Work out the finished part from the listing and answer in its coordinate system (mm). Coordinates: 2 decimals unless noted, no trailing zeros. Use one line per item in the form item = value.
from build123d import *

# Parameters (mm, degrees)
SKETCH_1_W      = 100
SKETCH_1_H      = 95
EXTRUDE_1_DEPTH = 2
HOLE_WIZARD_1_D = 3
FILLET_1_R      = 2


with BuildPart() as part:
    # 草图1 → 凸台-拉伸1 (new body)
    with BuildSketch(Plane(origin=(0, 0, 0), x_dir=(1, 0, 0), z_dir=(0, 1, 0))):
        Rectangle(SKETCH_1_W, SKETCH_1_H)
    extrude(amount=EXTRUDE_1_DEPTH)

    # 孔1 (through all)
    with Locations(Plane(origin=(0, 2, 0), x_dir=(1, 0, 0), z_dir=(0, 1, 0))):
        with Locations((-45, -12.906), (-42.5, 16.216), (42.673, 16.216), (45, -12.784)):
            Hole(HOLE_WIZARD_1_D / 2)

    # 圆角1
    fillet_1_edges = [part.edges().sort_by_distance(p)[0] for p in [
        (50, 1, 47.5),
        (-50, 1, 47.5),
        (-50, 1, -47.5),
        (50, 1, -47.5),
    ]]
    fillet(fillet_1_edges, radius=FILLET_1_R)


solid = part.part
(1) The mould has two halves that part along X. Classify faces 1 (the cylindrical face through (46.5, 0.99, 12.72)), 2 (the flat face through (-1, 0, -1)): released by +X, released by -X, zero draft, split by the parting line, or undercut.
Data:
face_1 = undercut
face_2 = zero draft
(2) Straight lines are drawn through the part: line 1 along X through (y, z) = (1.15, -16); line 2 along Z through (x, y) = (45, 0.5); line 3 along X through (y, z) = (0.5, 14). For each, find the intervals that lie inside material, in ascending order.
Data:
line_1 = -50 to -43.98, -41.02 to 41.19, 44.16 to 50
line_2 = -47.5 to 11.28, 14.28 to 47.5
line_3 = -50 to -46.03, -43.97 to 44.12, 45.88 to 50
(3) Each of these flat-tipped pins is pushed along its axis until it touches: P1, Ø1.5, axis at x = 24, z = -25.5, coming from the -Y side; P2, Ø1.8, axis at x = 45, z = 12.784, coming from the +Y side. Where does it stop, or does it pass through?
Data:
P1 = 0
P2 = through
